Input: part model. Units: mm. Frame: model coordinates. A direction names the side the tool comes from. Coordinates: 2 decimals unless noted, no trailing zeros. Loops run counter-clockwise (first coordinate to the right, second up) from the corner with the lowest first, then second, coordinate; pieces in that order, holes last.
(1) Section B-B, the plane z = 6. Return loops of the section in (x, y), then the cut area to 3 significant figures.
(2) Mould query, pull axis X, two halves, no side actions, for faces 1 (the face through (66, 0, 50)), 2 (the face through (0, 20, 50)), 3 (the face through (70, 20, 50)). Classes: released by +X, released by -X, zero draft, split by the parting line, or undercut.
(3) Line query: L1, parallel to X at y = 2, z = 61; L2, parallel to Y at x = 28.5, z = 91.5; L3, parallel to Y at x = 66, z = 45. Output: solid intervals per line, ascending.
(4) Section C-C, the plane x = 16. Return loops of the section in (y, z).
(5) Set-up query: faces 4 (the face through (66, -5, 52)), 5 (the face through (35, 46, 50)), 6 (the face through (3, 21, 50)). Return all of +Z, -Z, +X, -X, +Y, -Y with unobstructed straight access to the full face (end or side cutting, diameter ignored); none if empty.
(6) Contact query for flat-ended pins moving along their axis: P1, Ø12, axis at x = 57, y = 2.5, coming from the +Z side; P2, Ø5, axis at x = 59, z = 58, coming from the -Y side. Output: stop coordinate, or through.
(7) Section A-A, the plane y = 4. Return loops of the section in (x, z).
```python
from build123d import *

# Parameters (mm, degrees)
BOX002_W     = 6
BOX002_H     = 6
BOX002_DEPTH = 102
FILLET_R     = 5
BOX001_W     = 64
BOX001_H     = 43
BOX001_DEPTH = 102
BOX_W        = 70
BOX_H        = 46
BOX_DEPTH    = 102


with BuildPart() as fillet_body:
    # Box002 → Box002 (new body)
    with BuildSketch(Plane(origin=(0, -6, 0), x_dir=(1, 0, 0), z_dir=(0, 0, 1))):
        with Locations((3, 3)):
            Rectangle(BOX002_W, BOX002_H)
    extrude(amount=BOX002_DEPTH)

    # Fillet
    fillet_edges = [fillet_body.edges().sort_by_distance(p)[0] for p in [
        (6, -6, 51),
    ]]
    fillet(fillet_edges, radius=FILLET_R)


with BuildPart() as part_mirroring:
    # Part__Mirroring: instance of Fillet body
    add(fillet_body.part.mirror(Plane(origin=(0, 0, 0), x_dir=(0, -1, 0), z_dir=(1, 0, 0))))


with BuildPart() as part_mirroring_1:
    # Part__Mirroring placement: moved
    add(part_mirroring.part.moved(Location((70, 0, 0))))


with BuildPart() as box001:
    # Box001 → Box001 (new body)
    with BuildSketch(Plane(origin=(3, 0, 0), x_dir=(1, 0, 0), z_dir=(0, 0, 1))):
        with Locations((32, 21.5)):
            Rectangle(BOX001_W, BOX001_H)
    extrude(amount=BOX001_DEPTH)


with BuildPart() as fusion:
    # Box → Box (new body)
    with BuildSketch(Plane.XY):
        with Locations((35, 23)):
            Rectangle(BOX_W, BOX_H)
    extrude(amount=BOX_DEPTH)

    # Cut: cut Box001
    add(box001.part, mode=Mode.SUBTRACT)

    # Fusion: union Fillet body, Part__Mirroring
    add(fillet_body.part)
    add(part_mirroring_1.part)


solid = fusion.part
```
Report:
1. outline: (0, -6) - (1, -6) arc R5 ccw to (6, -1) - (6, 0) - (3, 0) - (3, 43) - (67, 43) - (67, 0) - (64, 0) - (64, -1) arc R5 ccw to (69, -6) - (70, -6) - (70, 46) - (0, 46) - close
1. area: 529 mm2
2. face 1: undercut
2. face 2: released by -X
2. face 3: released by +X
3. L1: x = 0 to 3, 67 to 70
3. L2: y = 43 to 46
3. L3: y = -5 to 0, 43 to 46
4. outline: (43, 0) - (46, 0) - (46, 102) - (43, 102) - close
5. face 4: +Z, -Z, -Y
5. face 5: +Z, -Z, +X, -X, +Y
5. face 6: +Z, -Z
6. P1: passes through
6. P2: stops at y = 43
7. outline: (0, 0) - (3, 0) - (3, 102) - (0, 102) - close; (67, 0) - (70, 0) - (70, 102) - (67, 102) - close
